from build123d import *

# Parameters (mm, degrees)
SKETCH1_W               = 8
SKETCH1_H               = 8
BOSS_EXTRUDE1_DEPTH     = 3
CUT_EXTRUDE1_DEPTH      = 12.704699911
CUT_EXTRUDE1_DEPTH_BACK = 12.704699911
CUT_EXTRUDE2_DEPTH      = 11
SKETCH4_R               = 1.8
CUT_EXTRUDE3_DEPTH      = 0.8
SKETCH5_W               = 8
SKETCH5_H               = 1
BOSS_EXTRUDE2_DEPTH     = 2
FILLET1_R               = 4
CUT_EXTRUDE4_DEPTH      = 0.4


with BuildPart() as part:
    # Sketch1 → Boss-Extrude1 (new body)
    with BuildSketch(Plane(origin=(0, 0, 0), x_dir=(1, 0, 0), z_dir=(0, 1, 0))):
        with Locations((4, 4)):
            Rectangle(SKETCH1_W, SKETCH1_H)
    extrude(amount=BOSS_EXTRUDE1_DEPTH)

    # Sketch2 → Cut-Extrude1 (cut, two sides: drawn at the far end of the back side and taken through both)
    with BuildSketch(Plane.XY.offset(-CUT_EXTRUDE1_DEPTH_BACK)):
        Polygon((0, 0), (0.6, 3), (0, 3), align=None)
        Polygon((8, 0), (7.4, 3), (8, 3), align=None)
    extrude(amount=CUT_EXTRUDE1_DEPTH + CUT_EXTRUDE1_DEPTH_BACK, mode=Mode.SUBTRACT)

    # Sketch3 → Cut-Extrude2 (cut)
    with BuildSketch(Plane(origin=(0, 0, 0), x_dir=(0, 0, -1), z_dir=(1, 0, 0))):
        Polygon((0, 0), (0.6, 3), (0, 3), align=None)
        Polygon((8, 3), (7.4, 3), (8, 0), align=None)
    extrude(amount=CUT_EXTRUDE2_DEPTH, mode=Mode.SUBTRACT)

    # Sketch4 → Cut-Extrude3 (cut)
    with BuildSketch(Plane.XZ):
        with Locations(Location((4, -3.75, 0), (0, 0, 270))):
            Circle(SKETCH4_R)
    extrude(amount=-CUT_EXTRUDE3_DEPTH, mode=Mode.SUBTRACT)

    # Sketch5 → Boss-Extrude2 (add)
    with BuildSketch(Plane.XZ):
        with Locations((4, -7.5)):
            Rectangle(SKETCH5_W, SKETCH5_H)
    extrude(amount=BOSS_EXTRUDE2_DEPTH)

    # Fillet1
    # the kernel refuses this fillet: 4 mm, written as the material it takes off along each edge
    with BuildSketch(Plane(origin=(8, -2, -16.660254038), x_dir=(0, 1, 0), z_dir=(0, 0, 1)), Plane(origin=(0, -2, 1.660254038), x_dir=(0, 1, 0), z_dir=(0, 0, -1))) as fillet1_piece_1:
        with BuildLine():
            CenterArc((4, 3.464101615), FILLET1_R, 180, 60)
            Line((0, 3.464101615), (-0.08, 3.464101615))
            Line((-0.08, 3.464101615), (-0.08, 0))
            Line((-0.08, 0), (0, -0.08))
            ThreePointArc((0, -0.08), (1, -0.08), (1.96, -0.069282032))
            Line((1.96, -0.069282032), (2, 0))
        make_face()
    extrude(amount=18.320508076, mode=Mode.SUBTRACT)

    # Sketch6 → Cut-Extrude4 (cut)
    with BuildSketch(Plane(origin=(0, 3, 0), x_dir=(1, 0, 0), z_dir=(0, 1, 0))):
        with BuildLine():
            Line((4.478635236, 6.002856352), (5.247866005, 6.002856352))
            Line((5.247866005, 6.002856352), (5.247866005, 3.481221736))
            add(Edge.make_bspline(
                [(5.247866005, 3.481221736), (5.247522255, 3.441153869), (5.246855206, 3.363401883), (5.242756502, 3.250390465), (5.236658321, 3.14454193), (5.227277222, 3.045871471), (5.21405872, 2.954592388), (5.200049867, 2.869976575), (5.183041427, 2.792451692), (5.167800036, 2.743951306), (5.160526262, 2.72080507)],
                knots=[0, 0, 0, 0, 1.251619961, 2.428777588, 3.532126049, 4.56323557, 5.523704531, 6.412540087, 7.242403515, 8, 8, 8, 8], degree=3))
            add(Edge.make_bspline(
                [(5.160526262, 2.72080507), (5.150361081, 2.692282601), (5.130243602, 2.635834988), (5.091141653, 2.555314881), (5.046176431, 2.479084315), (4.995474484, 2.406812938), (4.939514717, 2.338210987), (4.876399077, 2.275086649), (4.8083478, 2.215238098), (4.733446681, 2.161145289), (4.653580791, 2.110709794), (4.566475051, 2.068688963), (4.473843299, 2.032340387), (4.374908104, 2.002816628), (4.269640778, 1.979716073), (4.158311001, 1.962901894), (4.040770466, 1.95334773), (3.960490164, 1.952175274), (3.919340364, 1.9515743)],
                knots=[0, 0, 0, 0, 0.925533072, 1.831683394, 2.73255258, 3.630007683, 4.529542467, 5.436465751, 6.357118906, 7.298274949, 8.259461937, 9.242242071, 10.251058183, 11.300341426, 12.396409345, 13.544807631, 14.74152597, 16, 16, 16, 16], degree=3))
            add(Edge.make_bspline(
                [(3.919340364, 1.9515743), (3.871225528, 1.952737211), (3.777685944, 1.954998015), (3.641661475, 1.97000769), (3.514100564, 1.996260242), (3.395387048, 2.034179675), (3.284307874, 2.08131717), (3.182206561, 2.140114726), (3.088540477, 2.209392701), (3.003918711, 2.289363431), (2.928299433, 2.379218215), (2.863026475, 2.479745415), (2.80762712, 2.589893743), (2.762984692, 2.710161506), (2.727739397, 2.839972913), (2.702317462, 2.979601288), (2.687147894, 3.129126134), (2.684913172, 3.2319872), (2.683763441, 3.284907634)],
                knots=[0, 0, 0, 0, 1.114068574, 2.165849827, 3.164101702, 4.124467949, 5.046988974, 5.952942428, 6.846011651, 7.738523925, 8.642829306, 9.558838605, 10.50752403, 11.491963144, 12.524197802, 13.618364352, 14.774685164, 16, 16, 16, 16], degree=3))
            Line((2.683763441, 3.284907634), (3.45299421, 3.336189685))
            add(Edge.make_bspline(
                [(3.45299421, 3.336189685), (3.454375767, 3.307862598), (3.45702498, 3.25354382), (3.464380935, 3.175240866), (3.473682687, 3.103271277), (3.485853837, 3.037851064), (3.498960823, 2.978427444), (3.515987002, 2.926169857), (3.533886556, 2.879240769), (3.549608387, 2.851783511), (3.557160877, 2.838593531)],
                knots=[0, 0, 0, 0, 1.326609226, 2.543847584, 3.678365909, 4.719972403, 5.656527627, 6.521948534, 7.28997025, 8, 8, 8, 8], degree=3))
            add(Edge.make_bspline(
                [(3.557160877, 2.838593531), (3.56872297, 2.821148121), (3.59147861, 2.786813382), (3.632990929, 2.742071605), (3.677558537, 2.702955843), (3.727619554, 2.672203009), (3.781780527, 2.648016829), (3.840448037, 2.63044225), (3.903460331, 2.619785853), (3.946808463, 2.61876437), (3.969019851, 2.618240967)],
                knots=[0, 0, 0, 0, 1.023658308, 2.014687051, 2.979722519, 3.920049697, 4.880550909, 5.878122304, 6.912759386, 8, 8, 8, 8], degree=3))
            add(Edge.make_bspline(
                [(3.969019851, 2.618240967), (3.991477248, 2.618659453), (4.034647527, 2.619463917), (4.09686091, 2.626779219), (4.154063033, 2.638632824), (4.206285054, 2.655294856), (4.253703868, 2.676924623), (4.295268393, 2.704596166), (4.33276969, 2.735732915), (4.36516489, 2.773188264), (4.392766236, 2.818318957), (4.415812105, 2.873248962), (4.43563784, 2.938204221), (4.450960178, 3.01367855), (4.464002509, 3.098949399), (4.472183692, 3.194770716), (4.478064386, 3.300859295), (4.478439634, 3.37517575), (4.478635236, 3.413914044)],
                knots=[0, 0, 0, 0, 0.980314827, 1.884477813, 2.730827652, 3.527503874, 4.27366112, 4.998269146, 5.70163477, 6.396145331, 7.150281155, 8.001758491, 8.990432449, 10.111292654, 11.361572691, 12.75538406, 14.308707205, 16, 16, 16, 16], degree=3))
            Line((4.478635236, 3.413914044), (4.478635236, 6.002856352))
        make_face()
    extrude(amount=-CUT_EXTRUDE4_DEPTH, mode=Mode.SUBTRACT)


solid = part.part
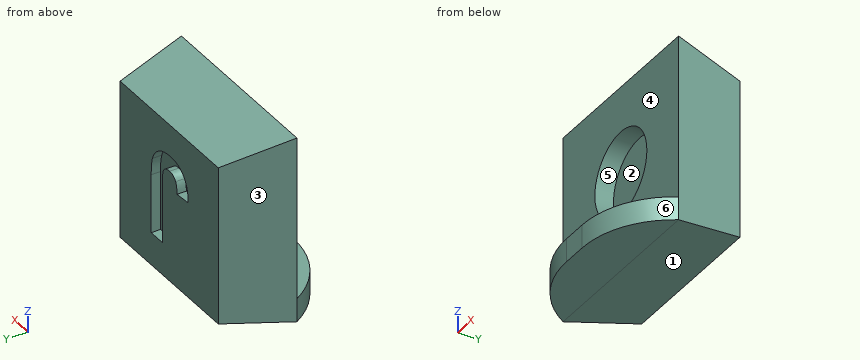
Here's how the part is built. I have some questions about the finished solid (model axes, mm). Face numbers are marked on the shaded views. A direction names the side the tool comes from. Give positions to 0.01 mm unless a question says otherwise; leave off trailing zeros. Loops run counter-clockwise (first coordinate to the right, second up) from the corner with the lowest first, then second, coordinate; pieces in that order, holes last. Notation, with made-up numbers: (86, 33.25) -> (120, 33.25) arc R7 cw to (120, 40.25) -> close; hole circle Ø6 at (-19, 88). An arc over 180 degrees is marked (long way). One line per item, written item: value.
Q1. If I drill on line 1 along Y through (x, z) = (3, -1.5); line 2 along Z through (x, y) = (3.25, -0.3); line 3 along X through (y, z) = (0.3, -3.75), over which ranges is the centre line in solid material (lowest first)?
Answers follow:
line 1: 0 to 3
line 2: -8 to -7
line 3: 0.06 to 2.2, 5.8 to 7.94
Q2. Suppose I cut it at A-A on z = -3.75. Please give me the cut outline in (x, y), then the cut area to 3 significant figures.
Answers follow:
outline: (0, 0) -> (2.2, 0) -> (2.2, 0.8) -> (5.8, 0.8) -> (5.8, 0) -> (8, 0) -> (7.4, 3) -> (5.25, 3) -> (5.25, 2.6) -> (4.48, 2.6) -> (4.48, 3) -> (0.6, 3) -> close
area: 19.0 mm^2
Q3. Suppose I cut it at D-D on z = -5. Please give me the cut outline in (x, y).
Answers follow:
outline: (0, 0) -> (2.7, 0) -> (2.7, 0.8) -> (5.3, 0.8) -> (5.3, 0) -> (8, 0) -> (7.4, 3) -> (5.25, 3) -> (5.25, 2.6) -> (4.48, 2.6) -> (4.48, 3) -> (0.6, 3) -> close
Q4. On a 3-axis mill with a long thin cutter (end or side, diameter ignored), from which of +Z, -Z, +X, -X, +Y, -Y can I reach the whole of each face in a straight line? I mean the marked faces 4, 5 and 6. Say none if no direction works.
Answers follow:
face 4: +Z, +X, -X, -Y
face 5: -Y
face 6: +Z, -Z, +X, -Y
Q5. Suppose I cut it at B-B on y = 0.65. Please give me the cut outline in (x, z).
Answers follow:
outline: (0.13, -7.87) -> (7.87, -7.87) -> (7.87, -0.13) -> (0.13, -0.13) -> close; hole circle Ø3.6 at (4, -3.75)
Q6. I'm going to push flat-ended pins straight in: pin 1 Ø2 at (y, z) = (2, -4.5) entering from -X; pin 2 Ø2 at (x, z) = (3.5, -2.5) entering from -Y. Where does each tip first touch, or does it pass through?
Answers follow:
pin 1: x = 0.2
pin 2: y = 0
Q7. We'd pull the mould along X, two halves only. Please class the marked faces 1, 2 and 3: pulls with the +X half, pulls with the -X half, needs draft (parallel to the pull), parting line crosses it, or undercut.
Answers follow:
face 1: needs draft
face 2: undercut
face 3: pulls with the -X half
Q8. Suppose I cut it at C-C on x = 6.5. Please give me the cut outline in (y, z).
Answers follow:
outline: (-1.48, -8) -> (0, -8) -> (3, -7.4) -> (3, -0.6) -> (0, 0) -> (0, -7) -> (-1.48, -7) -> close
